```python
from build123d import *

# Parameters (mm, degrees)
IZIM1_W                     = 259.05
IZIM1_H                     = 33
Y_KSEKLIK_EKSTR_ZYON1_DEPTH = 7
IZIM2_W                     = 30
IZIM2_H                     = 2
KES_EKSTR_ZYON1_DEPTH       = 291
KES_EKSTR_ZYON2_DEPTH       = 291


with BuildPart() as part:
    # Çizim1 → Yükseklik-Ekstrüzyon1 (new body)
    with BuildSketch(Plane(origin=(0, 0, 0), x_dir=(1, 0, 0), z_dir=(0, 1, 0))):
        Rectangle(IZIM1_W, IZIM1_H)
    extrude(amount=Y_KSEKLIK_EKSTR_ZYON1_DEPTH)

    # Çizim2 → Kes-Ekstrüzyon1 (cut)
    with BuildSketch(Plane(origin=(129.525, 0, 0), x_dir=(0, 0, -1), z_dir=(1, 0, 0))):
        with Locations((0, 6)):
            Rectangle(IZIM2_W, IZIM2_H)
    extrude(amount=-KES_EKSTR_ZYON1_DEPTH, mode=Mode.SUBTRACT)

    # Çizim3 → Kes-Ekstrüzyon2 (cut)
    with BuildSketch(Plane(origin=(129.525, 0, 0), x_dir=(0, 0, -1), z_dir=(1, 0, 0))):
        with BuildLine():
            Line((-15, 5), (15, 5))
            Line((15, 5), (9.382352941, 2.003921569))
            ThreePointArc((9.382352941, 2.003921569), (7.5, 1.533333333), (5.617647059, 2.003921569))
            Line((5.617647059, 2.003921569), (1.882352941, 3.996078431))
            ThreePointArc((1.882352941, 3.996078431), (0, 4.466666667), (-1.882352941, 3.996078431))
            Line((-1.882352941, 3.996078431), (-5.617647059, 2.003921569))
            ThreePointArc((-5.617647059, 2.003921569), (-7.5, 1.533333333), (-9.382352941, 2.003921569))
            Line((-9.382352941, 2.003921569), (-15, 5))
        make_face()
    extrude(amount=-KES_EKSTR_ZYON2_DEPTH, mode=Mode.SUBTRACT)


solid = part.part
```
Geometry: final body of the model. Coordinates: model frame, mm. A direction names the side the tool comes from. Round coordinates to 2 decimals unless told otherwise and drop trailing zeros. Order: outer loops, then holes, each group sorted by start corner. A loop starts at its lowest first (then second) coordinate and runs counter-clockwise, first axis right, second up. Notation, with made-up numbers: M -20.75,-28 L 31.25,-28 A20 cw 31.25,-24 Z; hole C 64,41.5 d1. An arc over 180 degrees is marked long. Use one line per item in the form item = value. Start each with the question number.
Q1. Mould query, pull axis Z, two halves, no side actions, for faces 1 (the face through (-2, 3, -16.5)), 2 (the face through (-2, 0, 0)), 3 (the face through (-2, 3, 16.5)), 4 (the face through (1.813, 3.523, -12.23)). Classes: +Z half, -Z half, draft (parallel to the pull), parting line (faces both ways), or undercut.
Q2. Material intervals for line 1 (Z direction, x = 69, y = 2); line 2 (Z direction, x = -91, y = 3.75); line 3 (Z direction, x = -91.5, y = 5.75), sorted ascending. Write a range as [from, to].
Q3. Cut plane A-A (x = -70). Return loops of the section in (y, z).
Q4. Pin query (flat end, axial travel): pin 1 Ø6 at (x, z) = (-25, 3.5) entering from +Y. Return the tip coordinate at first contact, or that it passes through.
Q5. Access query for faces 5 (the face through (129.525, 2, 0)), 6 (the face through (1.81, 3.48, 12.15)). Directions: +Z, -Z, +X, -X, +Y, -Y. A direction counts if a zero-diameter tool reaches every point of the face in a straight line with its end or side. Return the directions, or none.
Geometry results:
q1.face_1 = -Z half
q1.face_2 = draft
q1.face_3 = +Z half
q1.face_4 = undercut
q2.line_1 = [-16.5, -9.37], [-5.63, 5.63], [9.37, 16.5]
q2.line_2 = [-16.5, -12.66], [-2.34, 2.34], [12.66, 16.5]
q2.line_3 = [-16.5, -15], [15, 16.5]
q3.outline = M 0,-16.5 L 7,-16.5 L 7,-15 L 5,-15 L 2,-9.38 A4 cw 2,-5.62 L 4,-1.88 A4 ccw 4,1.88 L 2,5.62 A4 cw 2,9.38 L 5,15 L 7,15 L 7,16.5 L 0,16.5 Z
q4.pin_1 = 4.44
q5.face_5 = +Z, -Z, +X, +Y, -Y
q5.face_6 = +X, -X, +Y
